from build123d import *

# Parameters (mm, degrees)
SM_BASE_FLANGE_1_DEPTH = 65
CUT_EXTRUDE_1_DEPTH    = 82.547532152
PATTERN_LINEAR_1_COUNT = 2
PATTERN_LINEAR_1_PITCH = 45
CHAMFER_1_SIZE         = 5
CUT_EXTRUDE_2_DEPTH    = 82.547532152
SKETCH_8_R             = 2.1
CUT_EXTRUDE_3_DEPTH    = 82.547532152
PATTERN_LINEAR_2_COUNT = 2
PATTERN_LINEAR_2_PITCH = 45
FILLET_1_R             = 5


# Sheet-metal steps are written as plain solids
with BuildPart() as part:
    # Sketch 1 → 基材-凸緣1 (new body)
    with BuildSketch(Plane.XY):
        with BuildLine():
            Line((0, 45), (0, 0.7366))
            ThreePointArc((0, 0.7366), (-0.215745145, 0.215745145), (-0.7366, 0))
            Line((-0.7366, 0), (-20, 0))
            Line((-20, 0), (-20, -3))
            Line((-20, -3), (-0.7366, -3))
            ThreePointArc((-0.7366, -3), (1.905575199, -1.905575199), (3, 0.7366))
            Line((3, 0.7366), (3, 45))
            Line((3, 45), (0, 45))
        make_face()
    extrude(amount=SM_BASE_FLANGE_1_DEPTH)

    # 草圖6 → 除料-伸長1 (cut, through all)
    with BuildSketch(Plane(origin=(0, 0, 0), x_dir=(-1, 0, 0), z_dir=(0, 1, 0))):
        with BuildLine():
            Line((7.8683, 57.1), (12.8683, 57.1))
            ThreePointArc((12.8683, 57.1), (14.9683, 55), (12.8683, 52.9))
            Line((12.8683, 52.9), (7.8683, 52.9))
            ThreePointArc((7.8683, 52.9), (5.7683, 55), (7.8683, 57.1))
        make_face()
    cut_extrude_1 = extrude(amount=-CUT_EXTRUDE_1_DEPTH, mode=Mode.SUBTRACT)

    # 直線複製排列1: 除料-伸長1 ×2
    with Locations(*[(0, 0, -i * PATTERN_LINEAR_1_PITCH) for i in range(1, PATTERN_LINEAR_1_COUNT)]):
        add(cut_extrude_1, mode=Mode.SUBTRACT)

    # 導角1
    chamfer_1_edges = [part.edges().sort_by_distance(p)[0] for p in [
        (-20, -1.5, 65),
        (-20, -1.5, 0),
    ]]
    chamfer(chamfer_1_edges, length=CHAMFER_1_SIZE)

    # 草圖7 → 除料-伸長2 (cut, through all)
    with BuildSketch(Plane.ZY):
        Polygon((0, 45), (65, 45), (65, 35.864845744), align=None)
    extrude(amount=-CUT_EXTRUDE_2_DEPTH, mode=Mode.SUBTRACT)

    # 草圖8 → 除料-伸長3 (cut, through all)
    with BuildSketch(Plane.ZY):
        with Locations((8.510949678, 33.705588303)):
            Circle(SKETCH_8_R)
    cut_extrude_3 = extrude(amount=-CUT_EXTRUDE_3_DEPTH, mode=Mode.SUBTRACT)

    # 直線複製排列2: 除料-伸長3 ×2
    with Locations(*[Vector(0, -0.13917310096005842, 0.9902680687415713) * (i * PATTERN_LINEAR_2_PITCH) for i in range(1, PATTERN_LINEAR_2_COUNT)]):
        add(cut_extrude_3, mode=Mode.SUBTRACT)

    # 圓角1
    fillet_1_edges = [part.edges().sort_by_distance(p)[0] for p in [
        (1.5, 35.864845744, 65),
        (1.5, 45, 0),
    ]]
    fillet(fillet_1_edges, radius=FILLET_1_R)


solid = part.part
Work out the finished part from the listing and answer in its coordinate system (mm). A direction names the side the tool comes from. Give positions to 0.01 mm unless a question says otherwise; leave off trailing zeros. Order: outer loops, then holes, each group sorted by start corner. A loop starts at its lowest first (then second) coordinate and runs counter-clockwise, first axis right, second up. Notation, with made-up numbers: (29.5, 88.5) -> (62.5, 88.5) arc R29 ccw to (62.5, 126.5) -> close; hole circle Ø4 at (54.25, 78). An arc over 180 degrees is marked (long way). Answer as a JSON object with one key per item and string values. Group by question number.
1. Section B-B on z = 9 is taken. Determine the outline of the cut face in (x, y).
2. Flat-ended cylindrical pins translate along their axes: pin 1 Ø6 at (x, z) = (-14, 31.5) entering from +Y; pin 2 Ø3.5 at (y, z) = (27.44, 53.07) entering from +X; pin 3 Ø8 at (x, z) = (-0.5, 43.5) entering from +Y; pin 4 Ø2 at (y, z) = (35, 15.5) entering from -X. Find the tip coordinate at first contact, or state that the pin passes through.
3. Section C-C on z = 56 is taken. Determine the outline of the cut face in (x, y), plus the area to 3 significant figures.
4. The mould has two halves that part along X. Classify faces 1 (the cylindrical face through (1.88, -1.93, 32.04)), 2 (the flat face through (-10, -1, 7.9)), 3 (the cylindrical face through (1.479, 32.428, 6.844)), 4 (the flat face through (-10, -1, 12.1)): released by +X, released by -X, zero draft, split by the parting line, or undercut.
5. Section D-D on x = -15.75 is taken. Determine the outline of the cut face in (y, z), plus the area to 4 significant figures.
6. Section A-A on y = 26.5 is taken. Determine the outline of the cut face in (x, z).
7. A tool of negligible diameter and unlimited length cuts with its end or side. For faces 5 (the cylindrical face through (1.479, 27.535, 50.975)), 6 (the flat face through (-10, 0, 32)), 7 (the flat face through (-10, -1, 52.9)), from which of +Z, -Z, +X, -X, +Y, -Y can it reach the whole face along a straight path? Write none if from no direction.
8. Consider line 1 along X through (y, z) = (16, 51); line 2 along Y through (x, z) = (-4.25, 13); line 3 along Y through (x, z) = (2.25, 30.5). Determine where each line is inside the solid, lowest interval first. Write a range as [from, to].
Result sheet:
{
 "1": {"outline": "(-20, -3) -> (-14.71, -3) -> (-14.71, 0) -> (-20, 0) -> close; (-6.02, -3) -> (-0.74, -3) arc R3.74 ccw to (3, 0.74) -> (3, 31.66) -> (0, 31.66) -> (0, 0.74) arc R0.74 cw to (-0.74, 0) -> (-6.02, 0) -> close; (0, 35.75) -> (3, 35.75) -> (3, 43.74) -> (0, 43.74) -> close"},
 "2": {"pin 1": "stops at y = 0", "pin 2": "passes through", "pin 3": "stops at y = 39.44", "pin 4": "stops at x = 0"},
 "3": {"outline": "(-20, -3) -> (-14.71, -3) -> (-14.71, 0) -> (-20, 0) -> close; (-6.02, -3) -> (-0.74, -3) arc R3.74 ccw to (3, 0.74) -> (3, 37.13) -> (0, 37.13) -> (0, 0.74) arc R0.74 cw to (-0.74, 0) -> (-6.02, 0) -> close", "area": "151 mm^2"},
 "4": {"face 1": "released by +X", "face 2": "undercut", "face 3": "zero draft", "face 4": "undercut"},
 "5": {"outline": "(-3, 0.75) -> (0, 0.75) -> (0, 64.25) -> (-3, 64.25) -> close", "area": "190.5 mm^2"},
 "6": {"outline": "(0, 0) -> (3, 0) -> (3, 51.2) -> (0, 51.2) -> close; (0, 54.95) -> (3, 54.95) -> (3, 65) -> (0, 65) -> close"},
 "7": {"face 5": "+X, -X", "face 6": "+Z, -Z, -X, +Y", "face 7": "+Y, -Y"},
 "8": {"line 1": "x = [0, 3]", "line 2": "y = [-3, 0]", "line 3": "y = [-1.51, 40.71]"}
}
